Here's how the part is built. I have some questions about the finished solid (model axes, mm). Face numbers are marked on the shaded views. A direction names the side the tool comes from. Round coordinates to 2 decimals unless told otherwise and drop trailing zeros. Write each loop counter-clockwise with the first axis right and the second up, starting at its lowest first coordinate (ties: lowest second). Pieces come first, ordered by that corner, then holes. Notation, with made-up numbers: (51, 80.25) - (73, 80.25) arc R30 ccw to (73, 106.25) - close; hole circle Ø10 at (-15, -37). An arc over 180 degrees is marked (long way). One line per item, written item: value. Start each with the question number.
Item 1: Imagine slicing it at A-A, the plane z = -17. Please give me the cut outline in (x, y), then the cut area to 3 significant figures.
Item 2: For the marked faces 1, 2, 3, 4 and 5, which set-ups out of +Z, -Z, +X, -X, +Y, -Y let a thin tool reach every point of the face, with its end or its side?
Item 3: Imagine slicing it at B-B, the plane y = 5. Please give me the cut outline in (x, z).
Item 4: For P1, Ø12, axis at y = 23.5, z = 13.5, coming from the +X side; P2, Ø20, axis at y = 19.5, z = -9.5, coming from the -X side; P3, Ø1.5, axis at x = 63.5, y = 16.5, coming from the +Z side; P4, Ø4, axis at x = 48, z = 2.5, coming from the +Y side, each with a flat end and sliding along its axis, tell me the tip position at first contact or that it passes through.
Item 5: Imagine slicing it at C-C, the plane x = 1.5. Please give me the cut outline in (y, z), then the cut area to 3 significant figures.
Item 6: If I drill on line 1 (X direction, y = 16.5, z = 6.5); line 2 (X direction, y = 24, z = 4); line 3 (X direction, y = 21, z = 0.5), over which ranges is the centre line in solid material (lowest first)?
Item 7: Imagine slicing it at D-D, the plane z = 9.5. Please give me the cut outline in (x, y), then the cut area to 3 significant figures.
Item 8: Thinking about a two-plate mould opening in X: for the marked faces 6, 7, 8 and 9, which applies, released by +X, released by -X, zero draft, split by the parting line, or undercut?
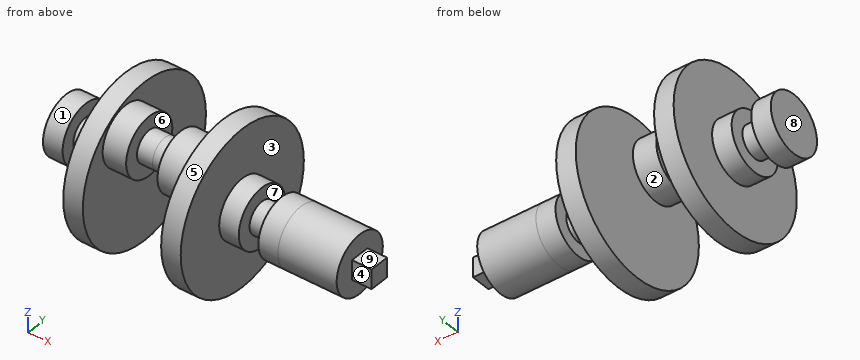
```python
from build123d import *

# Parameters (mm, degrees)
F0_R      = 20
F1_DEPTH  = 5
F3_R      = 7.5
F4_DEPTH  = 5
F5_R      = 4
F6_DEPTH  = 5
F7_R      = 7.5
F7_R_2    = 4
F8_DEPTH  = 5
F2_R      = 7.5
F9_DEPTH  = 6
F10_R     = 4
F11_DEPTH = 4
F13_R     = 7.5
F14_DEPTH = 15
F15_W     = 5
F15_H     = 5
F16_DEPTH = 5


with BuildPart() as f1:
    # F0 (on Right) → F1 (new body)
    with BuildSketch(Plane.YZ):
        with Locations((17.2490278537, 0)):
            Circle(F0_R)
    extrude(amount=F1_DEPTH)

    # F3 (on face) → F4 (join)
    with BuildSketch(Plane(origin=(0, 0, 0), x_dir=(0, -1, 0), z_dir=(-1, 0, 0))):
        with Locations((-17.2490278537, 0)):
            Circle(F3_R)
    extrude(amount=F4_DEPTH)

    # F5 (on face) → F6 (join)
    with BuildSketch(Plane(origin=(-5, 0, 0), x_dir=(0, -1, 0), z_dir=(-1, 0, 0))):
        with Locations((-17.2490278537, 0)):
            Circle(F5_R)
    extrude(amount=F6_DEPTH)

    # F7 (on face) → F8 (join)
    with BuildSketch(Plane(origin=(-10, 0, 0), x_dir=(0, -1, 0), z_dir=(-1, 0, 0))):
        with Locations((-17.2490278537, 0)):
            Circle(F7_R)
        with Locations((-17.2490278537, 0)):
            Circle(F7_R_2, mode=Mode.SUBTRACT)
        with Locations((-17.2490278537, 0)):
            Circle(F7_R_2)
    extrude(amount=F8_DEPTH)

    # F2 (on face) → F9 (join)
    with BuildSketch(Plane.YZ.offset(5)):
        with Locations((11.1903151186, 10.3581851689)):
            Circle(F2_R)
    extrude(amount=F9_DEPTH)

    # F10 (on face) → F11 (join)
    with BuildSketch(Plane.YZ.offset(11)):
        with Locations((11.1903151186, 10.3581851689)):
            Circle(F10_R)
    extrude(amount=F11_DEPTH)

    # F12: F1 across face


with BuildPart() as f1_1:
    add(f1.part)
    add(f1.part.mirror(Plane(origin=(15, 11.1903151186, 10.3581851689), x_dir=(0, 1, 0), z_dir=(1, 0, 0))))

    # F13 (on face) → F14 (join)
    with BuildSketch(Plane.YZ.offset(45)):
        with Locations((17.2490278537, 0)):
            Circle(F13_R)
    extrude(amount=F14_DEPTH)

    # F15 (on face) → F16 (join)
    with BuildSketch(Plane.YZ.offset(60)):
        with Locations((17.2490278537, 0)):
            Rectangle(F15_W, F15_H)
    extrude(amount=F16_DEPTH)


solid = f1_1.part
```
Values follow:
1. outline: (0, 6.71) - (5, 6.71) - (5, 27.78) - (0, 27.78) - close; (25, 6.71) - (30, 6.71) - (30, 27.78) - (25, 27.78) - close
1. area: 211 mm^2
2. face 1: -X
2. face 2: none
2. face 3: +X
2. face 4: +Z, -Z, +X, -Y
2. face 5: +X, -X
3. outline: (0, -15.81) - (5, -15.81) - (5, 6.12) - (11, 6.12) - (11, 14.59) - (5, 14.59) - (5, 15.81) - (0, 15.81) - close; (19, 6.12) - (25, 6.12) - (25, -15.81) - (30, -15.81) - (30, 15.81) - (25, 15.81) - (25, 14.59) - (19, 14.59) - close
4. P1: stops at x = 30
4. P2: stops at x = -15
4. P3: stops at z = 2.5
4. P4: stops at y = 24.73
5. outline: circle Ø40 at (17.25, 0)
5. area: 1,260 mm^2
6. line 1: x = -15 to -10, -5 to 11, 19 to 35, 40 to 60
6. line 2: x = 0 to 5, 25 to 30
6. line 3: x = -15 to 5, 25 to 60
7. outline: (0, -0.35) - (5, -0.35) - (5, 3.74) - (11, 3.74) - (11, 7.28) - (19, 7.28) - (19, 3.74) - (25, 3.74) - (25, -0.35) - (30, -0.35) - (30, 34.85) - (25, 34.85) - (25, 18.64) - (19, 18.64) - (19, 15.1) - (11, 15.1) - (11, 18.64) - (5, 18.64) - (5, 34.85) - (0, 34.85) - close
7. area: 593 mm^2
8. face 6: undercut
8. face 7: undercut
8. face 8: released by -X
8. face 9: zero draft
